Build history of the part. All positions in model axes, mm. A direction names the side the tool comes from. Round coordinates to 2 decimals unless told otherwise and drop trailing zeros. Loops run counter-clockwise (first coordinate to the right, second up) from the corner with the lowest first, then second, coordinate; pieces in that order, holes last. Notation, with made-up numbers: (39.5, -38.75) - (51.5, -38.75) arc R15 ccw to (51.5, -29.75) - close; hole circle Ø2 at (-40, 84.5). An arc over 180 degrees is marked (long way). One line per question, with ' | ' between items. Start each with the question number.
from build123d import *

# Parameters (mm, degrees)
SKETCH1_W                     = 75
SKETCH1_H                     = 130
BASE_FLANGE1_DEPTH            = 1.89738
EDGE_FLANGE1_STRIP_W          = 12.66952
EDGE_FLANGE1_STRIP_H          = 1.89738
EDGE_FLANGE1_STRIP_CUT_DEPTH  = 100
EDGE_FLANGE1_RELIEF_W         = 13.61821
EDGE_FLANGE1_RELIEF_H         = 0.94869
EDGE_FLANGE1_RELIEF_CUT_DEPTH = 1.89738
EDGE_FLANGE1_DEPTH            = 100
SKETCH18_R                    = 3
SKETCH18_R_2                  = 36.022471604
CUT_EXTRUDE1_DEPTH            = 10
BREAK_CORNER1_DEPTH           = 1.89738
BREAK_CORNER2_START           = -1.89738
BREAK_CORNER2_DEPTH           = 1.89738
CUT_EXTRUDE2_DEPTH            = 10
EDGE_FLANGE2_DEPTH            = 30
EDGE_FLANGE3_DEPTH            = 25.56262
EDGE_FLANGE4_DEPTH            = 30
EDGE_FLANGE5_DEPTH            = 25.56262
BREAK_CORNER3_START           = 38.678740931
BREAK_CORNER3_OUTLINE_W       = 18
BREAK_CORNER3_OUTLINE_H       = 1.89738
BREAK_CORNER3_DEPTH           = 7.071067812
BREAK_CORNER4_START           = 2.16
BREAK_CORNER4_DEPTH           = 1.89738
SKETCH32_W                    = 6.59738
SKETCH32_H                    = 15
CUT_EXTRUDE3_DEPTH            = 10


# Read off the part's stored shape, not the designer's step: Break-Corner1, Break-Corner2, Break-Corner3, Break-Corner4
# Sheet-metal steps are written as plain solids
with BuildPart() as part:
    # Sketch1 → Base-Flange1 (new body)
    with BuildSketch(Plane(origin=(0, 0, 0), x_dir=(1, 0, 0), z_dir=(0, 1, 0))):
        with Locations((37.5, 65)):
            Rectangle(SKETCH1_W, SKETCH1_H)
    extrude(amount=-BASE_FLANGE1_DEPTH)

    # Edge-Flange1 strip (across the edge) → Edge-Flange1 strip cut (cut)
    with BuildSketch(Plane.XY.offset(-115)):
        with Locations((-1.89738, -0.94869)):
            Rectangle(EDGE_FLANGE1_STRIP_W, EDGE_FLANGE1_STRIP_H)
    extrude(amount=EDGE_FLANGE1_STRIP_CUT_DEPTH, mode=Mode.SUBTRACT)

    # Edge-Flange1 relief (on the sheet) → Edge-Flange1 relief cut (cut)
    with BuildSketch(Plane(origin=(4.43738, 0, -115), x_dir=(1, 0, 0), z_dir=(0, 1, 0))):
        with Locations((-5.860415, 0.474345)):
            Rectangle(EDGE_FLANGE1_RELIEF_W, EDGE_FLANGE1_RELIEF_H)
        with Locations((-5.860415, -100.474345)):
            Rectangle(EDGE_FLANGE1_RELIEF_W, EDGE_FLANGE1_RELIEF_H)
    extrude(amount=-EDGE_FLANGE1_RELIEF_CUT_DEPTH, mode=Mode.SUBTRACT)

    # Edge-Flange1 section (across the edge) → Edge-Flange1 (add)
    with BuildSketch(Plane.XY.offset(-115)):
        with BuildLine():
            Line((0, 2.54), (0, 92))
            Line((0, 92), (1.89738, 92))
            Line((1.89738, 92), (1.89738, 2.54))
            ThreePointArc((1.89738, 2.54), (2.641328776, 0.743948776), (4.43738, 0))
            Line((4.43738, 0), (4.43738, -1.89738))
            ThreePointArc((4.43738, -1.89738), (1.299678511, -0.597701489), (0, 2.54))
        make_face()
    extrude(amount=EDGE_FLANGE1_DEPTH)

    # Sketch18 → Cut-Extrude1 (cut)
    with BuildSketch(Plane.ZY):
        with Locations(Location((-99.8, 85.14762, 0), (0, 0, 270))):
            Circle(SKETCH18_R)
        with Locations(Location((-30.2, 85.14762, 0), (0, 0, 270))):
            Circle(SKETCH18_R)
        with Locations(Location((-30.2, 15.54762, 0), (0, 0, 270))):
            Circle(SKETCH18_R)
        with Locations(Location((-99.8, 15.54762, 0), (0, 0, 270))):
            Circle(SKETCH18_R)
        with Locations(Location((-65, 50.34762, 0), (0, 0, 270))):
            Circle(SKETCH18_R_2)
    extrude(amount=-CUT_EXTRUDE1_DEPTH, mode=Mode.SUBTRACT)

    # Break-Corner1 outline → Break-Corner1 (cut)
    with BuildSketch(Plane.YZ):
        Polygon((92, -15), (82, -15), (92, -25), align=None)
        Polygon((92, -115), (92, -105), (82, -115), align=None)
    extrude(amount=BREAK_CORNER1_DEPTH, mode=Mode.SUBTRACT)

    # Break-Corner2 outline → Break-Corner2 (cut)
    with BuildSketch(Plane(origin=(0, 0, 0), x_dir=(1, 0, 0), z_dir=(0, 1, 0)).offset(BREAK_CORNER2_START)):
        Polygon((75, 130), (65, 130), (75, 120), align=None)
        Polygon((75, 0), (75, 10), (65, 0), align=None)
    extrude(amount=BREAK_CORNER2_DEPTH, mode=Mode.SUBTRACT)

    # Sketch19 → Cut-Extrude2 (cut)
    with BuildSketch(Plane(origin=(0, 0, 0), x_dir=(1, 0, 0), z_dir=(0, 1, 0))):
        with BuildLine():
            Line((60, 112), (20, 112))
            ThreePointArc((20, 112), (17, 115), (20, 118))
            Line((20, 118), (60, 118))
            ThreePointArc((60, 118), (63, 115), (60, 112))
        make_face()
        with BuildLine():
            Line((60, 12), (20, 12))
            ThreePointArc((20, 12), (17, 15), (20, 18))
            Line((20, 18), (60, 18))
            ThreePointArc((60, 18), (63, 15), (60, 12))
        make_face()
    extrude(amount=-CUT_EXTRUDE2_DEPTH, mode=Mode.SUBTRACT)

    # Edge-Flange2 section (across the edge) → Edge-Flange2 (add)
    with BuildSketch(Plane(origin=(6.59738, 0, 2.54), x_dir=(0, 0, -1), z_dir=(1, 0, 0))):
        with BuildLine():
            Line((-1.89738, 2.54), (-1.89738, 28.10262))
            Line((-1.89738, 28.10262), (0, 28.10262))
            Line((0, 28.10262), (0, 2.54))
            ThreePointArc((0, 2.54), (0.743948776, 0.743948776), (2.54, 0))
            Line((2.54, 0), (2.54, -1.89738))
            ThreePointArc((2.54, -1.89738), (-0.597701489, -0.597701489), (-1.89738, 2.54))
        make_face()
    extrude(amount=EDGE_FLANGE2_DEPTH)

    # Edge-Flange3 section (across the edge) → Edge-Flange3 (add)
    with BuildSketch(Plane(origin=(4.05738, 2.54, 2.54), x_dir=(1, 0, 0), z_dir=(0, 1, 0))):
        with BuildLine():
            Line((-1.89738, 2.54), (-1.89738, 23.10262))
            Line((-1.89738, 23.10262), (0, 23.10262))
            Line((0, 23.10262), (0, 2.54))
            ThreePointArc((0, 2.54), (0.743948776, 0.743948776), (2.54, 0))
            Line((2.54, 0), (2.54, -1.89738))
            ThreePointArc((2.54, -1.89738), (-0.597701489, -0.597701489), (-1.89738, 2.54))
        make_face()
    extrude(amount=EDGE_FLANGE3_DEPTH)

    # Edge-Flange4 section (across the edge) → Edge-Flange4 (add)
    with BuildSketch(Plane(origin=(36.59738, 0, -132.54), x_dir=(0, 0, 1), z_dir=(-1, 0, 0))):
        with BuildLine():
            Line((-1.89738, 2.54), (-1.89738, 28.10262))
            Line((-1.89738, 28.10262), (0, 28.10262))
            Line((0, 28.10262), (0, 2.54))
            ThreePointArc((0, 2.54), (0.743948776, 0.743948776), (2.54, 0))
            Line((2.54, 0), (2.54, -1.89738))
            ThreePointArc((2.54, -1.89738), (-0.597701489, -0.597701489), (-1.89738, 2.54))
        make_face()
    extrude(amount=EDGE_FLANGE4_DEPTH)

    # Edge-Flange5 section (across the edge) → Edge-Flange5 (add)
    with BuildSketch(Plane(origin=(4.05738, 28.10262, -132.54), x_dir=(1, 0, 0), z_dir=(0, -1, 0))):
        with BuildLine():
            Line((-1.89738, 2.54), (-1.89738, 23.10262))
            Line((-1.89738, 23.10262), (0, 23.10262))
            Line((0, 23.10262), (0, 2.54))
            ThreePointArc((0, 2.54), (0.743948776, 0.743948776), (2.54, 0))
            Line((2.54, 0), (2.54, -1.89738))
            ThreePointArc((2.54, -1.89738), (-0.597701489, -0.597701489), (-1.89738, 2.54))
        make_face()
    extrude(amount=EDGE_FLANGE5_DEPTH)

    # Break-Corner3 outline → Break-Corner3 (cut)
    with BuildSketch(Plane(origin=(0, 0, 0), x_dir=(0.707106781186548, -0.707106781186547, 0), z_dir=(0.707106781186547, 0.707106781186548, 0)).offset(BREAK_CORNER3_START)):
        with Locations((6, -3.48869)):
            Rectangle(BREAK_CORNER3_OUTLINE_W, BREAK_CORNER3_OUTLINE_H)
        with Locations((6, 133.48869)):
            Rectangle(BREAK_CORNER3_OUTLINE_W, BREAK_CORNER3_OUTLINE_H)
    extrude(amount=BREAK_CORNER3_DEPTH, mode=Mode.SUBTRACT)

    # Break-Corner4 outline → Break-Corner4 (cut)
    with BuildSketch(Plane.YZ.offset(BREAK_CORNER4_START)):
        Polygon((2.54, -20.56262), (7.54, -20.56262), (2.54, -15.56262), align=None)
        Polygon((28.10262, -15.56262), (23.10262, -20.56262), (28.10262, -20.56262), align=None)
        Polygon((28.10262, -109.43738), (23.10262, -109.43738), (28.10262, -114.43738), align=None)
        Polygon((2.54, -114.43738), (7.54, -109.43738), (2.54, -109.43738), align=None)
    extrude(amount=BREAK_CORNER4_DEPTH, mode=Mode.SUBTRACT)

    # Sketch32 → Cut-Extrude3 (cut)
    with BuildSketch(Plane(origin=(0, 0, 0), x_dir=(1, 0, 0), z_dir=(0, 1, 0))):
        with Locations((3.29869, 122.5)):
            Rectangle(SKETCH32_W, SKETCH32_H)
        with Locations((3.29869, 7.5)):
            Rectangle(SKETCH32_W, SKETCH32_H)
    extrude(amount=-CUT_EXTRUDE3_DEPTH, mode=Mode.SUBTRACT)


solid = part.part
1) Saw through at A-A on x = 41. Write the cut outline in (y, z).
2) Two-plate mould, pull along X, no slides. Class faces 6 (the cylindrical face through (63, -1, -115)), 7 (the flat face through (21, 15, 4.437)), 8 (the flat face through (0, 37, -99)): +X half, -X half, draft (parallel to the pull), parting line (faces both ways), or undercut.
3) Drop flat-ended pins along their axis: pin 1 (2 mm diameter, centred on x = 2.5, y = 44, fed in from -Z); pin 2 (5 mm diameter, centred on y = -0.5, z = -1, fed in from -X); pin 3 (12 mm diameter, centred on y = 9.5, z = -60.5, fed in from +X); pin 4 (7 mm diameter, centred on y = 15.55, z = -30.2, fed in from -X). Give the stop position or say it passes through.
4) Saw through at B-B on z = -92.5. Write the cut outline in (x, y), and give its area (3 significant figures).
5) Wall check: line 1 (X direction, y = 18, z = -81); line 2 (Y direction, x = 39, z = -54); line 3 (Z direction, x = 9.5, y = 6.5). Give the ranges that are in metal, low to high. Write a range as [from, to].
6) Saw through at D-D on y = 45. Write the cut outline in (x, z).
7) Tool access for faces 1 (the flat face through (39, -1.897, -66)), 2 (the cylindrical face through (17, -1, -115)), 3 (the flat face through (39, 0, -66)), 4 (the flat face through (36.597, 8, 3)), 5 (the flat face through (2.16, 16, -120)): list every direction of +Z, -Z, +X, -X, +Y, -Y with a clear straight run to the whole face (end or side of a thin tool).
8) Saw through at C-C on y = 76. Write the cut outline in (x, z), and give its area (3 significant figures).
Answer key:
1) outline: (-1.9, -130) - (0, -130) - (0, -118) - (-1.9, -118) - close; (-1.9, -112) - (0, -112) - (0, -18) - (-1.9, -18) - close; (-1.9, -12) - (0, -12) - (0, 0) - (-1.9, 0) - close
2) face 6: undercut | face 7: draft | face 8: -X half
3) pin 1: z = -115 | pin 2: x = 6.6 | pin 3: x = 1.9 | pin 4: x = 0
4) outline: (0, 2.54) arc R4.44 ccw to (4.44, -1.9) - (75, -1.9) - (75, 0) - (4.44, 0) arc R2.54 cw to (1.9, 2.54) - (1.9, 27.08) - (0, 27.08) - close; (0, 73.61) - (1.9, 73.61) - (1.9, 92) - (0, 92) - close | area: 226 mm²
5) line 1: [0, 1.9] | line 2: [-1.9, 0] | line 3: [-134.44, -132.54], [2.54, 4.44]
6) outline: (0, -115) - (1.9, -115) - (1.9, -100.62) - (0, -100.62) - close; (0, -29.38) - (1.9, -29.38) - (1.9, -15) - (0, -15) - close
7) face 1: +Z, -Z, +X, -X, -Y | face 2: +Y, -Y | face 3: +X, +Y | face 4: +Z, +X, +Y, -Y | face 5: +Z, -Z, +Y
8) outline: (0, -115) - (1.9, -115) - (1.9, -90.29) - (0, -90.29) - close; (0, -39.71) - (1.9, -39.71) - (1.9, -15) - (0, -15) - close | area: 93.8 mm²
